from build123d import *

# Parameters (mm, degrees)
SKETCH1_W           = 80
SKETCH1_H           = 20
BOSS_EXTRUDE1_DEPTH = 5
FILLET1_R           = 5
SHELL1_T            = -2
SKETCH3_W           = 6
SKETCH3_H           = 5
BOSS_EXTRUDE2_DEPTH = 6
SKETCH4_R           = 2
CUT_EXTRUDE1_DEPTH  = 4


with BuildPart() as part:
    # Sketch1 → Boss-Extrude1 (new body)
    with BuildSketch(Plane.XY):
        Rectangle(SKETCH1_W, SKETCH1_H)
    extrude(amount=BOSS_EXTRUDE1_DEPTH)

    # Fillet1
    fillet1_edges = [part.edges().sort_by_distance(p)[0] for p in [
        (-40, 10, 2.5),
        (40, 10, 2.5),
        (40, -10, 2.5),
        (-40, -10, 2.5),
    ]]
    fillet(fillet1_edges, radius=FILLET1_R)

    # Shell1
    shell1_openings = [part.faces().sort_by_distance(p)[0] for p in [
        (0, 0, 5),
    ]]
    offset(amount=SHELL1_T, openings=shell1_openings, kind=Kind.INTERSECTION)

    # Sketch3 → Boss-Extrude2 (add)
    with BuildSketch(Plane.XZ.offset(10)):
        with Locations((0, 2.5)):
            Rectangle(SKETCH3_W, SKETCH3_H)
    extrude(amount=BOSS_EXTRUDE2_DEPTH)

    # Sketch4 → Cut-Extrude1 (cut)
    with BuildSketch(Plane.XZ.offset(16)):
        with Locations((0, 2.5)):
            Circle(SKETCH4_R)
    extrude(amount=-CUT_EXTRUDE1_DEPTH, mode=Mode.SUBTRACT)


solid = part.part
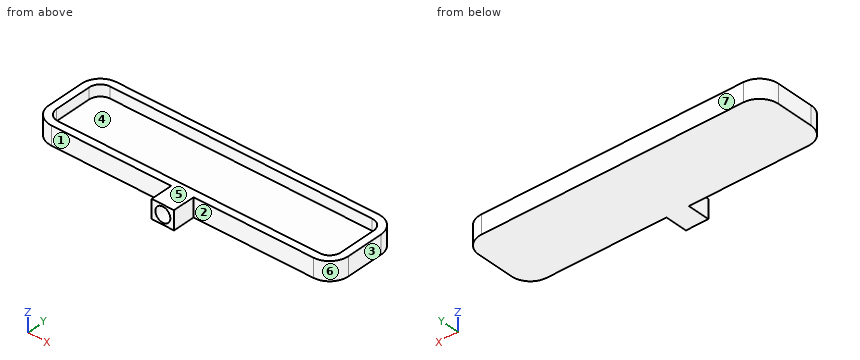
Model file for the job. Use its own axes, mm. Face numbers are marked on the shaded views. A direction names the side the tool comes from. Give positions to 0.01 mm unless a question says otherwise; leave off trailing zeros. Order: outer loops, then holes, each group sorted by start corner. A loop starts at its lowest first (then second) coordinate and runs counter-clockwise, first axis right, second up. Notation, with made-up numbers: (-9, 9.5) - (12, 9.5) arc R22 ccw to (12, 24.5) - close; hole circle Ø1 at (60.25, 84.5). An arc over 180 degrees is marked (long way). Return JSON: item names as keys, results as strings.
1) Flat gauge pins, fed straight in: P1, Ø1.5, axis at x = -24, y = 2.5, coming from the -Z side; P2, Ø1, axis at y = -8.5, z = 0.5, coming from the +X side; P3, Ø2.5, axis at x = 13.5, z = 3.5, coming from the -Y side; P4, Ø4, axis at x = 18, y = -4.5, coming from the +Z side. Where does each tip first touch, or does it go through?
Geometry says:
{"P1": "z = 0", "P2": "x = 39", "P3": "y = -10", "P4": "z = 2"}
2) Pull direction Y, two halves, no side cores. Call the marked faces 4, 5, 6 and 7: pulls with the +Y half, pulls with the -Y half, needs draft (parallel to the pull), parting line crosses it, or undercut.
Geometry says:
{"face 4": "undercut", "face 5": "needs draft", "face 6": "pulls with the -Y half", "face 7": "pulls with the +Y half"}
3) Cut at D-D, the plane x = 0. Give the cut face in (y, z), plus the area to 3 significant figures.
Geometry says:
{"outline": "(-16, 0) - (10, 0) - (10, 5) - (8, 5) - (8, 2) - (-8, 2) - (-8, 5) - (-16, 5) - (-16, 4.5) - (-12, 4.5) - (-12, 0.5) - (-16, 0.5) - close", "area": "66.0 mm²"}
4) Cut at C-C, the plane z = 3.35. Give the cut face in (x, y).
Geometry says:
{"outline": "(-40, -5) arc R5 ccw to (-35, -10) - (-3, -10) - (-3, -16) - (-1.81, -16) - (-1.81, -12) - (1.81, -12) - (1.81, -16) - (3, -16) - (3, -10) - (35, -10) arc R5 ccw to (40, -5) - (40, 5) arc R5 ccw to (35, 10) - (-35, 10) arc R5 ccw to (-40, 5) - close; hole (-38, -5) arc R3 ccw to (-35, -8) - (35, -8) arc R3 ccw to (38, -5) - (38, 5) arc R3 ccw to (35, 8) - (-35, 8) arc R3 ccw to (-38, 5) - close"}
5) Cut at A-A, the plane x = -10. Give the cut face in (y, z), plus the area to 3 significant figures.
Geometry says:
{"outline": "(-10, 0) - (10, 0) - (10, 5) - (8, 5) - (8, 2) - (-8, 2) - (-8, 5) - (-10, 5) - close", "area": "52.0 mm²"}
6) 3-axis set-ups, long thin cutter, end or side, ignore diameter. For the marked faces 1, 2 and 3: which of +Z, -Z, +X, -X, +Y, -Y reach the whole face in a straight line?
Geometry says:
{"face 1": "+Z, -Z, -X, -Y", "face 2": "+Z, -Z, +X, -Y", "face 3": "+Z, -Z, +X, +Y, -Y"}
7) Cut at B-B, the plane y = 2. Give the cut face in (x, z).
Geometry says:
{"outline": "(-40, 0) - (40, 0) - (40, 5) - (38, 5) - (38, 2) - (-38, 2) - (-38, 5) - (-40, 5) - close"}
8) Probe line 1 (Y direction, x = -9, z = 2.85); line 2 (Z direction, x = 0, y = -13.3); line 3 (X direction, y = 0.5, z = 2.45). List the from-to ranges inside material, lowest first. Write a range as from..to.
Geometry says:
{"line 1": "-10..-8, 8..10", "line 2": "0..0.5, 4.5..5", "line 3": "-40..-38, 38..40"}
